Here's the drawing with two shaded views (mm, measured from the low corner). I have some questions. A direction names the side the tool comes from. Coordinates: 2 decimals unless noted, no trailing zeros. Write each loop counter-clockwise with the first axis right and the second up, starting at its lowest first coordinate (ties: lowest second). Pieces come first, ordered by that corner, then holes. Notation, with made-up numbers: (48, 30.25) -> (90, 30.25) arc R31 ccw to (90, 66.25) -> close; hole circle Ø6 at (14.25, 49). An arc over 180 degrees is marked (long way). Put each result on its own line as item: value. Start each with the question number.
Item 1: I want a section at C-C, the plane x = 11. List the corners of the cut face in (y, z) for me, then the cut area to 3 significant figures.
Item 2: I need wall thicknesses on line 1 (X direction, y = 62.5, z = 45); line 2 (Y direction, x = 85.5, z = 34). Which ranges of each line are inside material? Lowest first, please. Write a range as [from, to].
Item 3: I want a section at A-A, the plane y = 19. List the corners of the cut face in (x, z) for me.
Item 4: If we mould it in two halves opening along X, with no side actions, what happens to the marked faces 1, 2 and 3? For each: released by +X, released by -X, zero draft, split by the parting line, or undercut.
Item 5: On a 3-axis mill with a long thin cutter (end or side, diameter ignored), from which of +Z, -Z, +X, -X, +Y, -Y can I reach the whole of each face in a straight line? I mean the marked faces 4 and 5. Say none if no direction works.
Item 6: I want a section at B-B, the plane z = 74. List the corners of the cut face in (x, y) for me, then the cut area to 3 significant figures.
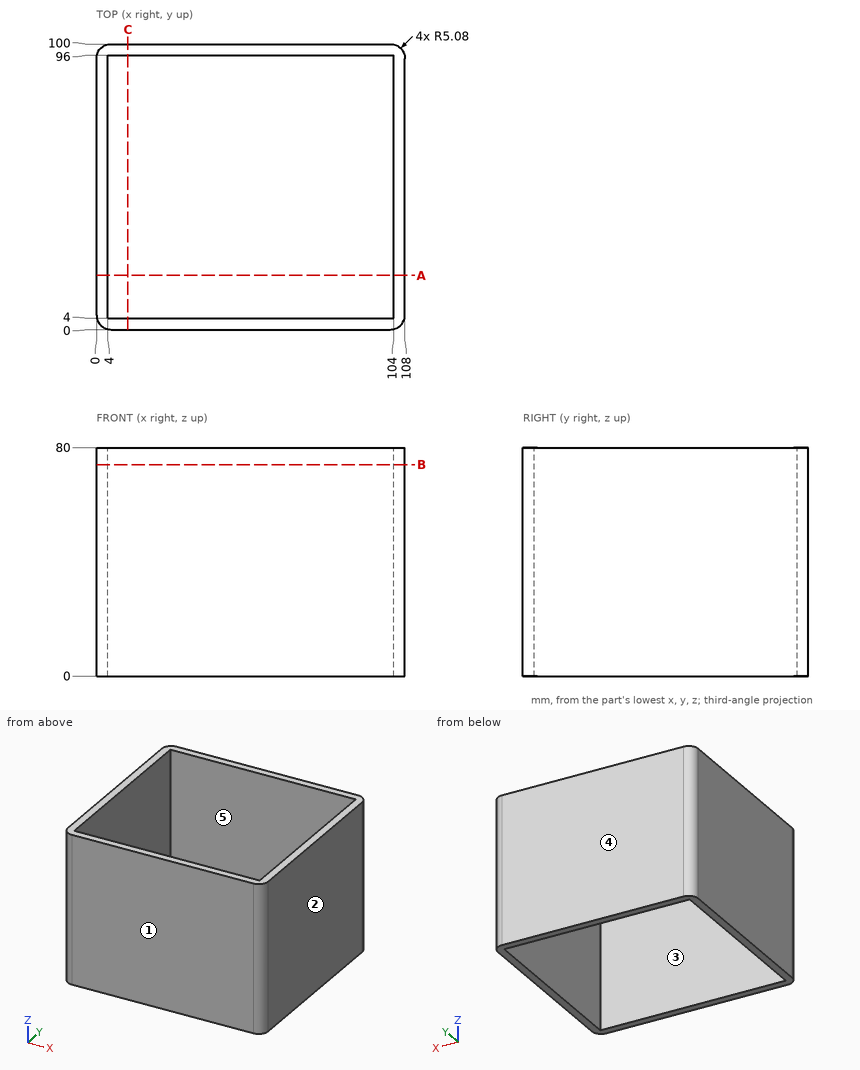
Calculated:
1. outline: (0, 0) -> (4, 0) -> (4, 80) -> (0, 80) -> close; (96, 0) -> (100, 0) -> (100, 80) -> (96, 80) -> close
1. area: 640 mm2
2. line 1: x = [0, 4], [104, 108]
2. line 2: y = [0, 4], [96, 100]
3. outline: (0, 0) -> (4, 0) -> (4, 80) -> (0, 80) -> close; (104, 0) -> (108, 0) -> (108, 80) -> (104, 80) -> close
4. face 1: zero draft
4. face 2: released by +X
4. face 3: undercut
5. face 4: +Z, -Z, +X, -X, +Y
5. face 5: +Z, -Z
6. outline: (0, 5.08) arc R5.08 ccw to (5.08, 0) -> (102.92, 0) arc R5.08 ccw to (108, 5.08) -> (108, 94.92) arc R5.08 ccw to (102.92, 100) -> (5.08, 100) arc R5.08 ccw to (0, 94.92) -> close; hole (4, 4) -> (104, 4) -> (104, 96) -> (4, 96) -> close
6. area: 1,580 mm2
